Geometry: final body of the model. Coordinates: model frame, mm. Face numbers are marked on the shaded views. Coordinates: 2 decimals unless noted, no trailing zeros. Order: outer loops, then holes, each group sorted by start corner. A loop starts at its lowest first (then second) coordinate and runs counter-clockwise, first axis right, second up. Notation, with made-up numbers: M 64.25,-13 L 115.25,-13 A18 cw 115.25,15 Z; hole C 1,34 d10. An arc over 180 degrees is marked long. One line per question, with ' | ' between items.
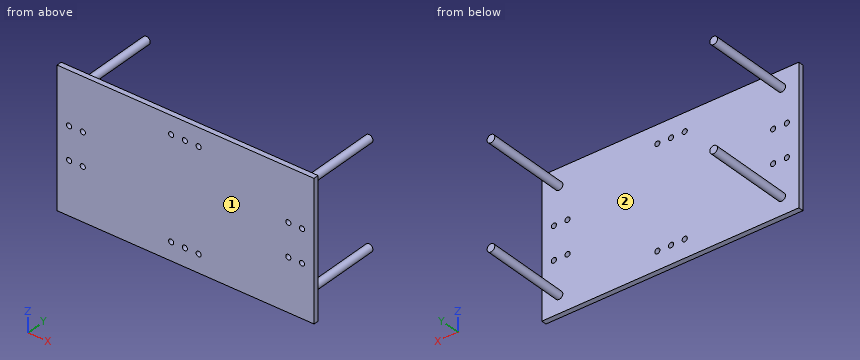
from build123d import *

# Parameters (mm, degrees)
SKETCH2_W           = 150
SKETCH2_H           = 80
SKETCH2_R           = 1.5
BOSS_EXTRUDE1_DEPTH = 3
SKETCH3_R           = 2.25
BOSS_EXTRUDE2_DEPTH = 50
SKETCH4_R           = 1.5
CUT_EXTRUDE1_DEPTH  = 10


with BuildPart() as part:
    # Sketch2 → Boss-Extrude1 (new body)
    with BuildSketch(Plane(origin=(0, 0, 0), x_dir=(1, 0, 0), z_dir=(0, 1, 0))):
        with Locations((-8.46473029, 1.825726141)):
            Rectangle(SKETCH2_W, SKETCH2_H)
        with Locations((-68.46473029, 11.325726141)):
            Circle(SKETCH2_R, mode=Mode.SUBTRACT)
        with Locations((-68.46473029, -7.674273859)):
            Circle(SKETCH2_R, mode=Mode.SUBTRACT)
        with Locations((-76.46473029, 11.325726141)):
            Circle(SKETCH2_R, mode=Mode.SUBTRACT)
        with Locations((-76.46473029, -7.674273859)):
            Circle(SKETCH2_R, mode=Mode.SUBTRACT)
        with Locations((51.53526971, -7.674273859)):
            Circle(SKETCH2_R, mode=Mode.SUBTRACT)
        with Locations((59.53526971, -7.674273859)):
            Circle(SKETCH2_R, mode=Mode.SUBTRACT)
        with Locations((59.53526971, 11.325726141)):
            Circle(SKETCH2_R, mode=Mode.SUBTRACT)
        with Locations((51.53526971, 11.325726141)):
            Circle(SKETCH2_R, mode=Mode.SUBTRACT)
    extrude(amount=-BOSS_EXTRUDE1_DEPTH)

    # Sketch3 → Boss-Extrude2 (add)
    with BuildSketch(Plane(origin=(0, 0, 0), x_dir=(1, 0, 0), z_dir=(0, 1, 0))):
        with Locations((56.53526971, 31.825726141)):
            Circle(SKETCH3_R)
        with Locations((56.53526971, -28.174273859)):
            Circle(SKETCH3_R)
        with Locations((-73.46473029, -28.174273859)):
            Circle(SKETCH3_R)
        with Locations((-73.46473029, 31.825726141)):
            Circle(SKETCH3_R)
    extrude(amount=BOSS_EXTRUDE2_DEPTH)

    # Sketch4 → Cut-Extrude1 (cut)
    with BuildSketch(Plane(origin=(0, -3, 0), x_dir=(-1, 0, 0), z_dir=(0, -1, 0))):
        with Locations((16.867382004, 31.325726141)):
            Circle(SKETCH4_R)
        with Locations((8.867382004, 31.325726141)):
            Circle(SKETCH4_R)
        with Locations((0.867382004, 31.325726141)):
            Circle(SKETCH4_R)
        with Locations((16.867382004, -27.674273859)):
            Circle(SKETCH4_R)
        with Locations((8.867382004, -27.674273859)):
            Circle(SKETCH4_R)
        with Locations((0.867382004, -27.674273859)):
            Circle(SKETCH4_R)
    extrude(amount=-CUT_EXTRUDE1_DEPTH, mode=Mode.SUBTRACT)


solid = part.part
1. Material intervals for line 1 (X direction, y = 18, z = 28.5); line 2 (Y direction, x = -25, z = 11.5); line 3 (X direction, y = 28.5, z = -31), sorted ascending. Write a range as [from, to].
Response values:
line 1: x = [-75.69, -71.24], [54.31, 58.76] | line 2: y = [-3, 0] | line 3: x = [-75.56, -71.37], [54.44, 58.63]
2. Draft query along Y for the marked faces 1 and 2. Return one class per face: pulls with the +Y half, pulls with the -Y half, needs draft (parallel to the pull), parting line crosses it, or undercut.
Response values:
face 1: pulls with the -Y half | face 2: pulls with the +Y half
3. Pin query (flat end, axial travel): P1, Ø4, axis at x = -16.87, z = 27.67, coming from the +Y side; P2, Ø4, axis at y = 7, z = 24.5, coming from the +X side; P3, Ø10, axis at y = 29.5, z = 28.5, coming from the -X side. Return the tip coordinate at first contact, or that it passes through.
Response values:
P1: stops at y = 0 | P2: stops at x = 58.04 | P3: stops at x = -75.71
4. Section A-A, the plane x = -53.5. Output: boundary loops of the cut face in (y, z), and give its area (3 significant figures).
Response values:
outline: M -3,-41.83 L 0,-41.83 L 0,38.17 L -3,38.17 Z | area: 240 mm^2
5. Section B-B, the plane y = 35. Output: boundary loops of the cut face in (x, z).
Response values:
outline: C -73.46,-31.83 d4.5; C -73.46,28.17 d4.5; C 56.54,-31.83 d4.5; C 56.54,28.17 d4.5
6. Section C-C, the plane z = 11. Output: boundary loops of the cut face in (x, y).
Response values:
outline: M -83.46,-3 L 66.54,-3 L 66.54,0 L -83.46,0 Z
